```python
from build123d import *

# Parameters (mm, degrees)
SKETCH1_W           = 9
SKETCH1_H           = 15
SKETCH1_W_2         = 15
SKETCH1_H_2         = 5
BOSS_EXTRUDE1_DEPTH = 12
SKETCH2_W           = 3.5
SKETCH2_H           = 12
CUT_EXTRUDE1_DEPTH  = 12
SKETCH3_W           = 20
SKETCH3_H           = 5
BOSS_EXTRUDE2_DEPTH = 5
SKETCH4_W           = 20
SKETCH4_H           = 5
BOSS_EXTRUDE3_DEPTH = 5
CHAMFER1_SIZE       = 1
FILLET1_R           = 1


with BuildPart() as part:
    # Sketch1 → Boss-Extrude1 (new body)
    with BuildSketch(Plane.XY):
        Rectangle(SKETCH1_W, SKETCH1_H)
        with Locations((-12, -5)):
            Rectangle(SKETCH1_W_2, SKETCH1_H_2)
        with Locations((12, -5)):
            Rectangle(SKETCH1_W_2, SKETCH1_H_2)
    extrude(amount=BOSS_EXTRUDE1_DEPTH)

    # Sketch2 → Cut-Extrude1 (cut)
    with BuildSketch(Plane(origin=(0, 7.5, 0), x_dir=(1, 0, 0), z_dir=(0, 1, 0))):
        with Locations((-0.05, -6)):
            Rectangle(SKETCH2_W, SKETCH2_H)
    extrude(amount=-CUT_EXTRUDE1_DEPTH, mode=Mode.SUBTRACT)

    # Sketch3 → Boss-Extrude2 (add)
    with BuildSketch(Plane.ZY.offset(19.5)):
        with Locations((6, -5)):
            Rectangle(SKETCH3_W, SKETCH3_H)
    extrude(amount=-BOSS_EXTRUDE2_DEPTH)

    # Sketch4 → Boss-Extrude3 (add)
    with BuildSketch(Plane(origin=(19.5, 0, 0), x_dir=(0, 0, -1), z_dir=(1, 0, 0))):
        with Locations((-6, -5)):
            Rectangle(SKETCH4_W, SKETCH4_H)
    extrude(amount=-BOSS_EXTRUDE3_DEPTH)

    # Chamfer1
    chamfer1_edges = [part.edges().sort_by_distance(p)[0] for p in [
        (-1.8, 1.5, 12),
        (-1.8, 1.5, 0),
        (1.7, 1.5, 0),
        (1.7, 1.5, 12),
        (-1.8, 7.5, 6),
        (1.7, 7.5, 6),
    ]]
    chamfer(chamfer1_edges, length=CHAMFER1_SIZE)

    # Fillet1
    fillet1_edges = [part.edges().sort_by_distance(p)[0] for p in [
        (9.5, -2.5, 0),
        (-9.5, -2.5, 0),
        (-4.5, 2.5, 0),
        (4.5, 2.5, 0),
        (-4.5, 2.5, 12),
        (4.5, -2.5, 6),
        (19.5, -2.5, 6),
        (-19.5, -2.5, 6),
        (-4.5, -2.5, 6),
        (-9.5, -2.5, 12),
        (9.5, -2.5, 12),
        (-14.5, -2.5, -2),
        (4.5, 2.5, 12),
        (-17, -2.5, -4),
        (-14.5, -2.5, 14),
        (-17, -2.5, 16),
        (14.5, -2.5, -2),
        (14.5, -2.5, 14),
        (17, -2.5, 16),
        (17, -2.5, -4),
    ]]
    fillet(fillet1_edges, radius=FILLET1_R)


solid = part.part
```
For this review, take the finished solid that the model builds, in its own axes (mm). A direction names the side the tool comes from. Round coordinates to 2 decimals unless told otherwise and drop trailing zeros. Write each loop counter-clockwise with the first axis right and the second up, starting at its lowest first coordinate (ties: lowest second). Pieces come first, ordered by that corner, then holes. Notation, with made-up numbers: (7, 48) - (36, 48) arc R30 ccw to (36, 85) - close; hole circle Ø7 at (0, 20). An arc over 180 degrees is marked (long way). Put each result on its own line as item: value.
Q1. Mouldability with a two-part tool opening along X and no side actions: class faces 5 (the face through (-4.801, -2.215, 6.07)), 6 (the face through (0, -4.5, 6)), 7 (the face through (4.785, -2.199, 6.07)), 8 (the face through (-14.5, -5, 14)) as released by +X, released by -X, zero draft, split by the parting line, or undercut.
Solved:
face 5: released by -X
face 6: undercut
face 7: released by +X
face 8: undercut
Q2. We need section D-D (x = 6). Give the boundary of the cut face in (y, z).
Solved:
outline: (-7.5, 0) - (-3.5, 0) arc R1 ccw to (-2.5, 1) - (-2.5, 11) arc R1 ccw to (-3.5, 12) - (-7.5, 12) - close
Q3. Machinability: for faces 1 (the face through (2.2, 7, 6.1)), 2 (the face through (4.199, 3.063, 11.715)), 3 (the face through (-4.5, 3, 6)), 4 (the face through (14.801, -2.785, 13.465)), which of the approach directions +Z, -Z, +X, -X, +Y, -Y give a long, thin tool a straight path to every point of the face, cutting with its end or side? Answer none if there is none.
Solved:
face 1: +Z, -Z, +Y
face 2: +Z, +X, +Y
face 3: +Z, -Z, -X, +Y
face 4: +Z, +Y
Q4. Insertion check: pin 1 Ø3 at (x, z) = (0.5, 7.5) entering from +Y; pin 2 Ø5 at (x, y) = (-7, -4.5) entering from -Z; pin 3 Ø7 at (y, z) = (5, 5.5) entering from -X. Each pin has a flat end and moves straight along its axis. Give the tip position at first contact, or say it passes through.
Solved:
pin 1: stops at y = 6.8
pin 2: stops at z = 0
pin 3: stops at x = -4.5
Q5. Wall thickness on probe 1 along X at (y, z) = (-1.25, 5); probe 2 along X at (y, z) = (-4, 2); probe 3 along Y at (x, z) = (10, 5.5): over which ranges is each line inside the solid? List them lowest first.
Solved:
probe 1: x = -4.5 to -1.8, 1.7 to 4.5
probe 2: x = -19.5 to -1.8, 1.7 to 19.5
probe 3: y = -7.5 to -2.5
Q6. We need section C-C (z = 1.5). Give the boundary of the cut face in (x, y).
Solved:
outline: (-19.5, -7.5) - (19.5, -7.5) - (19.5, -3.5) arc R1 ccw to (18.5, -2.5) - (5.5, -2.5) arc R1 cw to (4.5, -1.5) - (4.5, 7.5) - (2.7, 7.5) - (1.7, 6.5) - (1.7, -4.5) - (-1.8, -4.5) - (-1.8, 6.5) - (-2.8, 7.5) - (-4.5, 7.5) - (-4.5, -1.5) arc R1 cw to (-5.5, -2.5) - (-18.5, -2.5) arc R1 ccw to (-19.5, -3.5) - close
Q7. We need section B-B (z = -1.75). Give the boundary of the cut face in (x, y).
Solved:
outline: (-19.5, -7.5) - (-14.5, -7.5) - (-14.5, -3.5) arc R1 ccw to (-15.5, -2.5) - (-18.5, -2.5) arc R1 ccw to (-19.5, -3.5) - close; (14.5, -7.5) - (19.5, -7.5) - (19.5, -3.5) arc R1 ccw to (18.5, -2.5) - (15.5, -2.5) arc R1 ccw to (14.5, -3.5) - close
Q8. We need section A-A (y = 5). Give the boundary of the cut face in (x, z).
Solved:
outline: (-4.5, 1) arc R1 ccw to (-3.5, 0) - (-2.8, 0) - (-1.8, 1) - (-1.8, 11) - (-2.8, 12) - (-3.5, 12) arc R1 ccw to (-4.5, 11) - close; (1.7, 1) - (2.7, 0) - (3.5, 0) arc R1 ccw to (4.5, 1) - (4.5, 11) arc R1 ccw to (3.5, 12) - (2.7, 12) - (1.7, 11) - close
